Read the model definition and answer for the solid it produces. Units are mm, in the model's axes. Face numbers are marked on the shaded views. A direction names the side the tool comes from. Round coordinates to 2 decimals unless told otherwise and drop trailing zeros. Loops run counter-clockwise (first coordinate to the right, second up) from the corner with the lowest first, then second, coordinate; pieces in that order, holes last. Notation, with made-up numbers: (-8.5, -21.5) -> (14.5, -21.5) arc R7 cw to (14.5, -8.5) -> close; hole circle Ø4 at (85, 53.25). An arc over 180 degrees is marked (long way). Put each result on its own line as item: value.
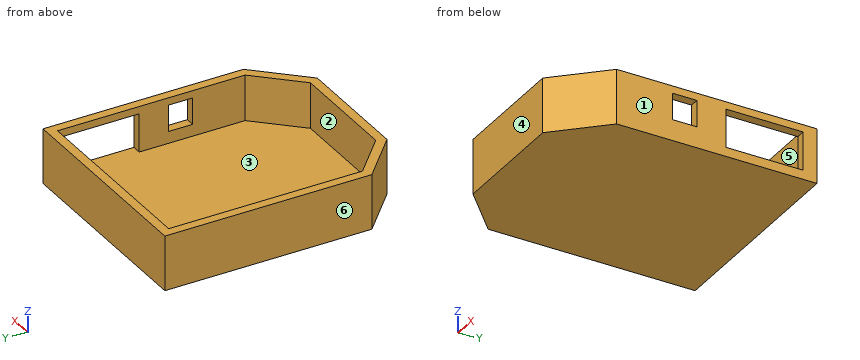
from build123d import *

# Parameters (mm, degrees)
F2_DEPTH = 5
F4_DEPTH = 25
F5_W     = 42
F5_H     = 21
F5_W_2   = 13.2
F5_H_2   = 14.5
F6_DEPTH = 5
F7_DEPTH = 5


with BuildPart() as f2:
    # F0 (on Top) → F2 (new body)
    with BuildSketch(Plane.XY):
        Polygon((28.673304, 123.177742), (-85.826696, 123.177742), (-85.826696, 10.177742), (-61.326696, -12.322258), (4.173304, -12.322258), (28.673304, 13.772988), align=None)
    extrude(amount=-F2_DEPTH)

    # F3 (on face) → F4 (join)
    with BuildSketch(Plane.XY):
        Polygon((4.173304, -12.322258), (28.673304, 13.772988), (28.673304, 123.177742), (-85.826696, 123.177742), (-85.826696, 10.177742), (-61.326696, -12.322258), align=None)
        Polygon((-80.826696, 118.177742), (23.673304, 118.177742), (23.673304, 15.75233), (2.009304, -7.322258), (-59.37912, -7.322258), (-80.826696, 12.374496), align=None, mode=Mode.SUBTRACT)
    extrude(amount=F4_DEPTH)

    # F5 (on face) → F6 (cut)
    with BuildSketch(Plane.YZ.offset(28.673304)):
        with Locations((94.577742, 10.5)):
            Rectangle(F5_W, F5_H)
        with Locations((50.977742, 13.75)):
            Rectangle(F5_W_2, F5_H_2)
    extrude(amount=F6_DEPTH, mode=Mode.SUBTRACT)

    # F5 (on face) → F7 (cut, through all)
    with BuildSketch(Plane.YZ.offset(28.673304)):
        with Locations((94.577742, 10.5)):
            Rectangle(F5_W, F5_H)
        with Locations((50.977742, 13.75)):
            Rectangle(F5_W_2, F5_H_2)
    extrude(amount=-F7_DEPTH, mode=Mode.SUBTRACT)


solid = f2.part
Item 1: Find the intervals of material crossed by line 1 along Y through (x, z) = (-55.5, 16); line 2 along X through (y, z) = (43, 23); line 3 along Z through (x, y) = (20.5, 35), in increasing order.
Derived:
line 1: y = -12.32 to -7.32, 118.18 to 123.18
line 2: x = -85.83 to -80.83, 23.67 to 28.67
line 3: z = -5 to 0
Item 2: Flat-ended cylindrical pins translate along their axes: pin 1 Ø6 at (x, y) = (11.5, 28.5) entering from +Z; pin 2 Ø1.5 at (x, z) = (27, 13.5) entering from -Y; pin 3 Ø4 at (x, z) = (27.5, 11.5) entering from -Y. Find the tip coordinate at first contact, or state that the pin passes through.
Derived:
pin 1: stops at z = 0
pin 2: stops at y = 11.19
pin 3: stops at y = 10.39
Item 3: For a pull along Y with two mould halves and no side action, classify the marked faces 1, 2, 3 and 4 as pulls with the +Y half, pulls with the -Y half, needs draft (parallel to the pull), parting line crosses it, or undercut.
Derived:
face 1: needs draft
face 2: undercut
face 3: undercut
face 4: pulls with the -Y half
Item 4: Which of the six approach directions +Z, -Z, +X, -X, +Y, -Y give full straight-line access (tool end or side, diameter ignored) to the marked faces 5 and 6?
Derived:
face 5: +Z
face 6: +Z, -Z, -X, +Y, -Y
Item 5: The part is cut by section D-D (z = 2). Determine the outline of the cut face in (x, y), then the cut area to 3 significant figures.
Derived:
outline: (-85.83, 10.18) -> (-61.33, -12.32) -> (4.17, -12.32) -> (28.67, 13.77) -> (28.67, 73.58) -> (23.67, 73.58) -> (23.67, 15.75) -> (2.01, -7.32) -> (-59.38, -7.32) -> (-80.83, 12.37) -> (-80.83, 118.18) -> (23.67, 118.18) -> (23.67, 115.58) -> (28.67, 115.58) -> (28.67, 123.18) -> (-85.83, 123.18) -> close
area: 2,060 mm^2
Item 6: The part is cut by section C-C (x = -20). Determine the outline of the cut face in (y, z), then the cut area to 4 significant figures.
Derived:
outline: (-12.32, -5) -> (123.18, -5) -> (123.18, 25) -> (118.18, 25) -> (118.18, 0) -> (-7.32, 0) -> (-7.32, 25) -> (-12.32, 25) -> close
area: 927.5 mm^2
Item 7: The part is cut by section A-A (y = 55.5). Determine the outline of the cut face in (x, z), then the cut area to 3 significant figures.
Derived:
outline: (-85.83, -5) -> (28.67, -5) -> (28.67, 6.5) -> (23.67, 6.5) -> (23.67, 0) -> (-80.83, 0) -> (-80.83, 25) -> (-85.83, 25) -> close; (23.67, 21) -> (28.67, 21) -> (28.67, 25) -> (23.67, 25) -> close
area: 750 mm^2
Item 8: The part is cut by section B-B (z = 11.5). Determine the outline of the cut face in (x, y).
Derived:
outline: (-85.83, 10.18) -> (-61.33, -12.32) -> (4.17, -12.32) -> (28.67, 13.77) -> (28.67, 44.38) -> (23.67, 44.38) -> (23.67, 15.75) -> (2.01, -7.32) -> (-59.38, -7.32) -> (-80.83, 12.37) -> (-80.83, 118.18) -> (23.67, 118.18) -> (23.67, 115.58) -> (28.67, 115.58) -> (28.67, 123.18) -> (-85.83, 123.18) -> close; (23.67, 57.58) -> (28.67, 57.58) -> (28.67, 73.58) -> (23.67, 73.58) -> close
